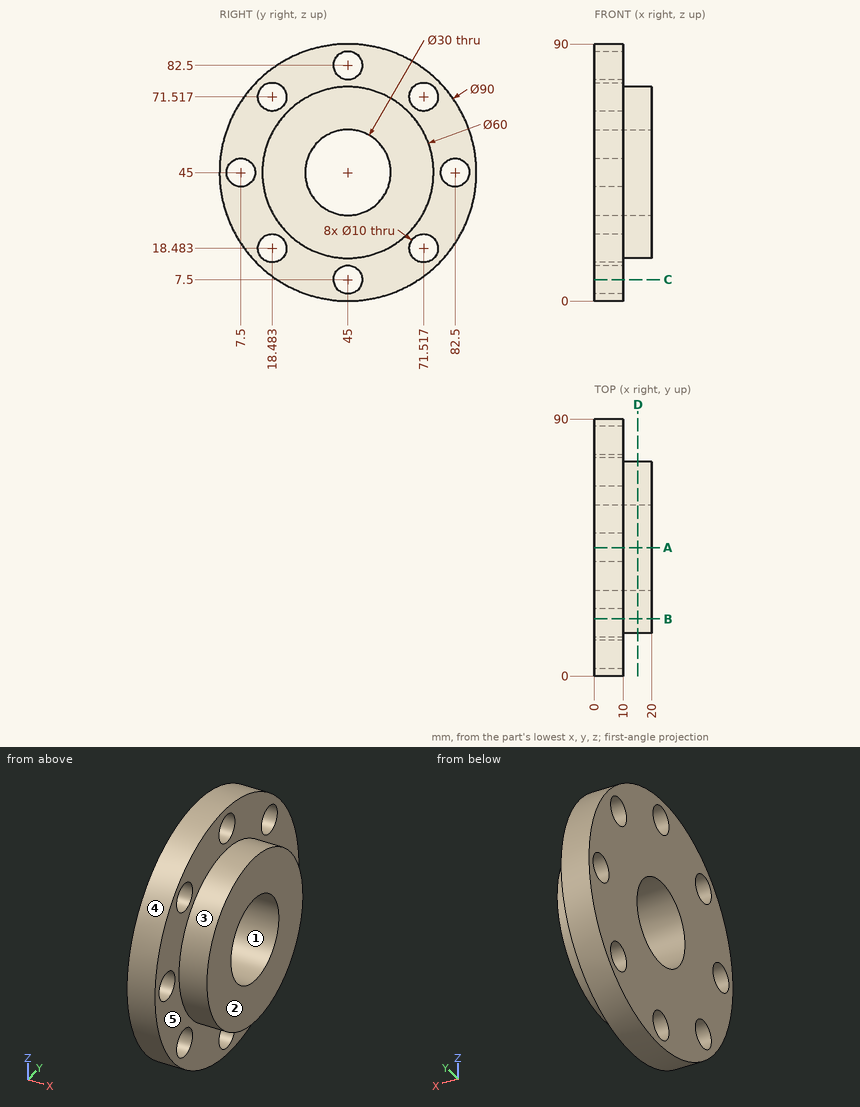
Geometry check sheet. Reference: drawing and pictorial views, mm from the part's lowest x, y, z. A direction names the side the tool comes from. Coordinates: 2 decimals unless noted, no trailing zeros. Loops run counter-clockwise (first coordinate to the right, second up) from the corner with the lowest first, then second, coordinate; pieces in that order, holes last.
1) Sectioned sample at D-D (x = 15.25). Record the boundary of the cut face in (y, z), and give its area (3 significant figures).
2) Sectioned sample at B-B (y = 20). Record the boundary of the cut face in (x, z).
3) Sectioned sample at A-A (y = 45). Record the boundary of the cut face in (x, z), and give its area (3 significant figures).
4) Release check for a two-part mould opening along Z. For the marked faces 1, 2 and 3 record: released by +Z, released by -Z, zero draft, split by the parting line, or undercut.
5) Material ranges on probe 1 along Z at (x, y) = (3.5, 46); probe 2 along Z at (x, y) = (6, 67.5) (1 decimal); probe 3 along Z at (x, y) = (6, 48) (1 decimal), recorded low to high.
6) Access from +Z, -Z, +X, -X, +Y, -Y to the whole of each face (thin tool, end or side, straight path). Record for the marked faces 4 and 5.
7) Sectioned sample at C-C (z = 7.5). Record the boundary of the cut face in (x, y) (1 decimal).
8) Gauge pin test, flat ends, axial feed: pin 1 (8 mm diameter, centred on x = 3, z = 33, fed in from +Y); pin 2 (18 mm diameter, centred on y = 45, z = 45, fed in from +X); pin 3 (6 mm diameter, centred on x = 4.5, z = 70.5, fed in from +Y); pin 4 (3 mm diameter, centred on x = 10, z = 31, fed in from +Y). Record the tip position at first contact, or that the pin passes through.
Check sheet entries:
1. outline: circle Ø60 at (45, 45); hole circle Ø30 at (45, 45)
1. area: 2,120 mm2
2. outline: (0, 7.58) - (10, 7.58) - (10, 13.72) - (0, 13.72) - close; (0, 23.25) - (10, 23.25) - (10, 28.42) - (20, 28.42) - (20, 61.58) - (10, 61.58) - (10, 66.75) - (0, 66.75) - close; (0, 76.28) - (10, 76.28) - (10, 82.42) - (0, 82.42) - close
3. outline: (0, 0) - (10, 0) - (10, 2.5) - (0, 2.5) - close; (0, 12.5) - (10, 12.5) - (10, 15) - (20, 15) - (20, 30) - (0, 30) - close; (0, 60) - (20, 60) - (20, 75) - (10, 75) - (10, 77.5) - (0, 77.5) - close; (0, 87.5) - (10, 87.5) - (10, 90) - (0, 90) - close
3. area: 700 mm2
4. face 1: undercut
4. face 2: zero draft
4. face 3: split by the parting line
5. probe 1: z = 0.01 to 2.6, 12.4 to 30.03, 59.97 to 77.6, 87.4 to 89.99
5. probe 2: z = 6 to 15.5, 21.5 to 68.5, 74.5 to 84
5. probe 3: z = 0.1 to 3.5, 11.5 to 30.3, 59.7 to 78.5, 86.5 to 89.9
6. face 4: +X, -X
6. face 5: +X
7. outline: (0, 20.1) - (10, 20.1) - (10, 40) - (0, 40) - close; (0, 50) - (10, 50) - (10, 69.9) - (0, 69.9) - close
8. pin 1: stops at y = 89.28
8. pin 2: passes through
8. pin 3: stops at y = 83.97
8. pin 4: stops at y = 88.23
